```python
from build123d import *

# Parameters (mm, degrees)
SKETCH1_R           = 28
BOSS_EXTRUDE1_DEPTH = 53
SKETCH2_R           = 16
BOSS_EXTRUDE2_DEPTH = 2
SKETCH3_R           = 6
BOSS_EXTRUDE3_DEPTH = 26
SKETCH4_W           = 57
SKETCH4_H           = 57
BOSS_EXTRUDE4_DEPTH = 60


with BuildPart() as part:
    # Sketch1 → Boss-Extrude1 (new body)
    with BuildSketch(Plane(origin=(0, 0, 0), x_dir=(1, 0, 0), z_dir=(0, 1, 0))):
        with Locations(Location((0, 0, 0), (0, 0, 270))):
            Circle(SKETCH1_R)
    extrude(amount=BOSS_EXTRUDE1_DEPTH)

    # Sketch2 → Boss-Extrude2 (add)
    with BuildSketch(Plane(origin=(0, 53, 0), x_dir=(1, 0, 0), z_dir=(0, 1, 0))):
        with Locations(Location((0, 0, 0), (0, 0, 270))):
            Circle(SKETCH2_R)
    extrude(amount=BOSS_EXTRUDE2_DEPTH)

    # Sketch3 → Boss-Extrude3 (add)
    with BuildSketch(Plane(origin=(0, 55, 0), x_dir=(1, 0, 0), z_dir=(0, 1, 0))):
        with Locations(Location((0, 0, 0), (0, 0, 90))):
            Circle(SKETCH3_R)
    extrude(amount=BOSS_EXTRUDE3_DEPTH)

    # Sketch4 → Boss-Extrude4 (add)
    with BuildSketch(Plane.XZ):
        Rectangle(SKETCH4_W, SKETCH4_H)
    extrude(amount=BOSS_EXTRUDE4_DEPTH)


solid = part.part
```
Geometry: final body of the model. Coordinates: model frame, mm. A direction names the side the tool comes from. Give positions to 0.01 mm unless a question says otherwise; leave off trailing zeros. Order: outer loops, then holes, each group sorted by start corner. A loop starts at its lowest first (then second) coordinate and runs counter-clockwise, first axis right, second up. Notation, with made-up numbers: M 64.5,55 L 79.5,55 A31 cw 79.5,89 Z; hole C 45.25,74.5 d8. An arc over 180 degrees is marked long. Answer as CSV lines item,"result". Start each with the question number.
1) Line query: line 1 (Y direction, x = 14, z = -5.5); line 2 (Y direction, x = 1, z = 22); line 3 (X direction, y = 52, z = 22). Output: solid intervals per line, ascending. Write a range as from..to.
2) Cut plane C-C (y = 51). Output: boundary loops of the cut face in (x, z).
3) Cut plane D-D (z = 10). Output: boundary loops of the cut face in (x, y), then the cut area to 3 significant figures.
4) Cut plane A-A (z = 0). Output: boundary loops of the cut face in (x, y).
5) Set-up query: faces 1 (the cylindrical face through (-27.334, 26.129, -6.07)), 2 (the flat face through (-28.5, -30, 0)). Return all of +Z, -Z, +X, -X, +Y, -Y with unobstructed straight access to the full face (end or side cutting, diameter ignored); none if empty.
6) First-contact query: P1, Ø5, axis at x = -12.5, z = 4, coming from the +Y side; P2, Ø3, axis at y = 20.5, z = -10.5, coming from the -X side; P3, Ø12, axis at x = -10.5, y = 36, coming from the +Z side. Flat tips, straight axial feed; report the tip coordinate or a pass-through.
7) Cut plane B-B (x = 0). Output: boundary loops of the cut face in (y, z).
Findings below:
1,line 1,"y = -60..55"
1,line 2,"y = -60..53"
1,line 3,"x = -17.32..17.32"
2,outline,"C 0,0 d56"
3,outline,"M -28.5,-60 L 28.5,-60 L 28.5,0 L 26.15,0 L 26.15,53 L 12.49,53 L 12.49,55 L -12.49,55 L -12.49,53 L -26.15,53 L -26.15,0 L -28.5,0 Z"
3,area,"6,240 mm²"
4,outline,"M -28.5,-60 L 28.5,-60 L 28.5,0 L 28,0 L 28,53 L 16,53 L 16,55 L 6,55 L 6,81 L -6,81 L -6,55 L -16,55 L -16,53 L -28,53 L -28,0 L -28.5,0 Z"
5,face 1,"+Y"
5,face 2,"+Z, -Z, -X, +Y, -Y"
6,P1,"stops at y = 55"
6,P2,"stops at x = -26.51"
6,P3,"stops at z = 27.64"
7,outline,"M -60,-28.5 L 0,-28.5 L 0,-28 L 53,-28 L 53,-16 L 55,-16 L 55,-6 L 81,-6 L 81,6 L 55,6 L 55,16 L 53,16 L 53,28 L 0,28 L 0,28.5 L -60,28.5 Z"
